The listing builds one solid part. Answer for the finished solid, in the listing's coordinates (mm). Round coordinates to 2 decimals unless told otherwise and drop trailing zeros. Order: outer loops, then holes, each group sorted by start corner. A loop starts at its lowest first (then second) coordinate and runs counter-clockwise, first axis right, second up. Notation, with made-up numbers: (-24.5, 82) - (34.5, 82) arc R27 cw to (34.5, 111) - close; hole circle Ø5 at (-18.5, 38.25). An arc over 180 degrees is marked (long way). Write item = value, one per line.
from build123d import *

# Parameters (mm, degrees)
SKETCH2_W                         = 647.7
SKETCH2_H                         = 12.7
BOSS_EXTRUDE1_DEPTH               = 52.07
CUT_EXTRUDE1_DEPTH                = 9.525
F_1_4_20_THREADED_HOLE_AT_2_COUNT = 2
F_1_4_20_THREADED_HOLE_AT_2_PITCH = 25.4
F_1_4_20_THREADED_HOLE_AT_3_COUNT = 2
F_1_4_20_THREADED_HOLE_AT_3_PITCH = 50.8
CUT_EXTRUDE2_DEPTH                = 329.255079778


with BuildPart() as part:
    # Sketch2 → Boss-Extrude1 (new, symmetric)
    with BuildSketch(Plane.XY):
        with Locations((0, -6.35)):
            Rectangle(SKETCH2_W, SKETCH2_H)
    extrude(amount=BOSS_EXTRUDE1_DEPTH, both=True)

    # Sketch3 → Cut-Extrude1 (cut)
    with BuildSketch(Plane(origin=(0, 0, 0), x_dir=(1, 0, 0), z_dir=(0, 1, 0))):
        with BuildLine():
            Line((63.675, 45.72), (-63.675, 45.72))
            ThreePointArc((-63.675, 45.72), (-65.796320344, 44.841320344), (-66.675, 42.72))
            Line((-66.675, 42.72), (-66.675, -42.72))
            ThreePointArc((-66.675, -42.72), (-65.796320344, -44.841320344), (-63.675, -45.72))
            Line((-63.675, -45.72), (63.675, -45.72))
            ThreePointArc((63.675, -45.72), (65.796320344, -44.841320344), (66.675, -42.72))
            Line((66.675, -42.72), (66.675, 42.72))
            ThreePointArc((66.675, 42.72), (65.796320344, 44.841320344), (63.675, 45.72))
        make_face()
    extrude(amount=-CUT_EXTRUDE1_DEPTH, mode=Mode.SUBTRACT)

    # Sketch6 → 1/4"-20 threaded hole (revolve, cut)
    with BuildSketch(Plane(origin=(-323.85, -6.35, -25.4), x_dir=(0, 0, 1), z_dir=(0, 1, 0))):
        Polygon((0, 0), (0, 52.707732465), (3.175, 50.8), (3.175, 0), align=None)
    f_1_4_20_threaded_hole = revolve(axis=Axis((-330.2, -6.35, -25.4), (1, 0, 0)), mode=Mode.SUBTRACT)

    # 1/4"-20 threaded hole at 2: 1/4"-20 threaded hole ×2
    with Locations(*[(0, 0, i * F_1_4_20_THREADED_HOLE_AT_2_PITCH) for i in range(1, F_1_4_20_THREADED_HOLE_AT_2_COUNT)]):
        add(f_1_4_20_threaded_hole, mode=Mode.SUBTRACT)

    # 1/4"-20 threaded hole at 3: 1/4"-20 threaded hole ×2
    with Locations(*[(0, 0, i * F_1_4_20_THREADED_HOLE_AT_3_PITCH) for i in range(1, F_1_4_20_THREADED_HOLE_AT_3_COUNT)]):
        add(f_1_4_20_threaded_hole, mode=Mode.SUBTRACT)

    # Mirror1: 1/4"-20 threaded hole across plane
    add(f_1_4_20_threaded_hole.mirror(Plane(origin=(0, 0, 0), x_dir=(0, 0, 1), z_dir=(1, 0, 0))), mode=Mode.SUBTRACT)

    # Mirror1 copy 1 sketch → Mirror1 copy 1 (revolve, cut)
    with BuildSketch(Plane(origin=(323.85, -6.35, 0), x_dir=(0, 0, 1), z_dir=(0, 1, 0))):
        Polygon((0, 0), (0, -52.707732465), (3.175, -50.8), (3.175, 0), align=None)
    revolve(axis=Axis((330.2, -6.35, 0), (1, 0, 0)), mode=Mode.SUBTRACT)

    # Mirror1 copy 2 sketch → Mirror1 copy 2 (revolve, cut)
    with BuildSketch(Plane(origin=(323.85, -6.35, 25.4), x_dir=(0, 0, 1), z_dir=(0, 1, 0))):
        Polygon((0, 0), (0, -52.707732465), (3.175, -50.8), (3.175, 0), align=None)
    revolve(axis=Axis((330.2, -6.35, 25.4), (1, 0, 0)), mode=Mode.SUBTRACT)

    # Sketch3<3> → Cut-Extrude2 (cut, through all)
    with BuildSketch(Plane(origin=(0, 0, 0), x_dir=(1, 0, 0), z_dir=(0, 1, 0))):
        with BuildLine():
            Line((57.325, 39.37), (-57.325, 39.37))
            ThreePointArc((-57.325, 39.37), (-59.446320344, 38.491320344), (-60.325, 36.37))
            Line((-60.325, 36.37), (-60.325, -36.37))
            ThreePointArc((-60.325, -36.37), (-59.446320344, -38.491320344), (-57.325, -39.37))
            Line((-57.325, -39.37), (57.325, -39.37))
            ThreePointArc((57.325, -39.37), (59.446320344, -38.491320344), (60.325, -36.37))
            Line((60.325, -36.37), (60.325, 36.37))
            ThreePointArc((60.325, 36.37), (59.446320344, 38.491320344), (57.325, 39.37))
        make_face()
    extrude(amount=-CUT_EXTRUDE2_DEPTH, mode=Mode.SUBTRACT)


solid = part.part
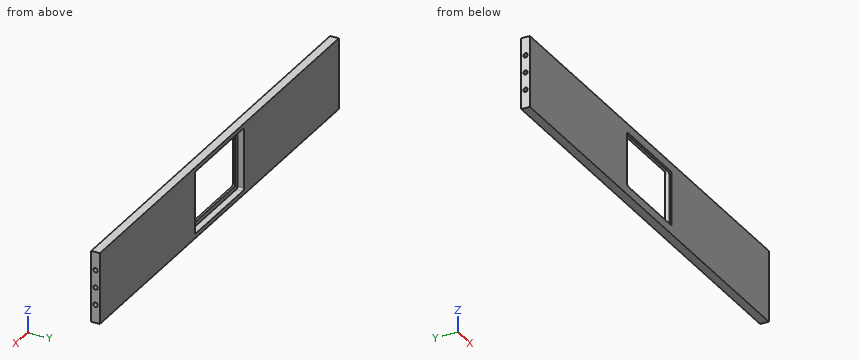
Q1. Find the intervals of material crossed by line 1 (Z direction, x = 295, y = -6.35) (3 decimals); line 2 (X direction, y = -11.5, z = 4.5) (3 decimals); line 3 (Y direction, x = -295, z = -25.4) (3 decimals), in increasing order. Write a range as from..to.
Model answer:
line_1 = -52.07..-28.575, -22.225..-3.175, 3.175..22.225, 28.575..52.07
line_2 = -323.85..-60.325, 60.325..323.85
line_3 = -12.7..-9.525, -3.175..0
Q2. Section A-A on x = -44.5 is taken. Determine the outline of the cut face in (y, z) (3 decimals), then the cut area to 3 significant figures.
Model answer:
outline = (-12.7, -52.07) - (0, -52.07) - (0, -45.72) - (-9.525, -45.72) - (-9.525, -39.37) - (-12.7, -39.37) - close; (-12.7, 39.37) - (-9.525, 39.37) - (-9.525, 45.72) - (0, 45.72) - (0, 52.07) - (-12.7, 52.07) - close
area = 202 mm^2
Q3. Flat-ended cylindrical pins translate along their axes: P1, Ø5.5, axis at y = -6.35, z = -25.4, coming from the +X side; P2, Ø5, axis at y = -6.35, z = 25.4, coming from the -X side; P3, Ø5, axis at x = 39.5, z = -40, coming from the +Y side (3 decimals). Find the tip coordinate at first contact, or state that the pin passes through.
Model answer:
P1 = 272.79
P2 = -272.64
P3 = -9.525
Q4. Section B-B on x = -281 is taken. Determine the outline of the cut face in (y, z) (3 decimals), then the cut area to 3 significant figures.
Model answer:
outline = (-12.7, -52.07) - (0, -52.07) - (0, 52.07) - (-12.7, 52.07) - close; hole circle Ø6.35 at (-6.35, -25.4); hole circle Ø6.35 at (-6.35, 0); hole circle Ø6.35 at (-6.35, 25.4)
area = 1,230 mm^2
